Work out the finished part from the listing and answer in its coordinate system (mm). Coordinates: 2 decimals unless noted, no trailing zeros. Write each loop counter-clockwise with the first axis right and the second up, starting at its lowest first coordinate (ties: lowest second). Pieces come first, ordered by that corner, then holes. Notation, with made-up numbers: M 67.5,-26.75 L 97.5,-26.75 A33 cw 97.5,11.25 Z; hole C 39.5,-1.75 d5. An arc over 180 degrees is marked long. Use CSV: the item, a comma, the result in double quotes.
from build123d import *

# Parameters (mm, degrees)
BOSS_EXTRUDE1_DEPTH        = 1.6
F_3_2_3_2_DIAMETER_HOLE3_D = 3.2
FILLET1_R                  = 2


with BuildPart() as part:
    # Sketch1 → Boss-Extrude1 (new body)
    with BuildSketch(Plane.XY):
        with BuildLine():
            Line((-84.56534388, -2.04814307), (-16.56534388, -2.04814307))
            Line((-16.56534388, -2.04814307), (-16.56534388, 7.95185693))
            Line((-16.56534388, 7.95185693), (-6.56534388, 7.95185693))
            Line((-6.56534388, 7.95185693), (-6.56534388, 3.95185693))
            Line((-6.56534388, 3.95185693), (3.425708931, 3.95185693))
            Line((3.425708931, 3.95185693), (3.43465612, 3.95185693))
            ThreePointArc((3.43465612, 3.95185693), (5.555976464, 4.830536587), (6.43465612, 6.95185693))
            Line((6.43465612, 6.95185693), (6.43465612, 88.95185693))
            ThreePointArc((6.43465612, 88.95185693), (5.555976464, 91.073177274), (3.43465612, 91.95185693))
            Line((3.43465612, 91.95185693), (-64.56534388, 91.95185693))
            Line((-64.56534388, 91.95185693), (-64.56534388, 81.95185693))
            Line((-64.56534388, 81.95185693), (-74.56534388, 81.95185693))
            Line((-74.56534388, 81.95185693), (-74.56534388, 85.95185693))
            Line((-74.56534388, 85.95185693), (-84.56534388, 85.95185693))
            ThreePointArc((-84.56534388, 85.95185693), (-86.686664224, 85.073177274), (-87.56534388, 82.95185693))
            Line((-87.56534388, 82.95185693), (-87.56534388, 0.95185693))
            ThreePointArc((-87.56534388, 0.95185693), (-86.686664224, -1.169463413), (-84.56534388, -2.04814307))
        make_face()
    extrude(amount=BOSS_EXTRUDE1_DEPTH)

    # Ø3.2 (3.2) Diameter Hole3 (through all)
    with Locations(Plane(origin=(0, 0, 0), x_dir=(-1, 0, 0), z_dir=(0, 0, -1))):
        with Locations((78.56534388, 6.95185693), (78.56534388, 82.95185693), (2.56534388, 82.95185693), (2.56534388, 6.95185693)):
            Hole(F_3_2_3_2_DIAMETER_HOLE3_D / 2)

    # Fillet1
    fillet1_edges = [part.edges().sort_by_distance(p)[0] for p in [
        (-16.56534388, 7.95185693, 0.8),
        (-74.56534388, 81.95185693, 0.8),
        (-64.56534388, 81.95185693, 0.8),
        (-6.56534388, 7.95185693, 0.8),
    ]]
    fillet(fillet1_edges, radius=FILLET1_R)


solid = part.part
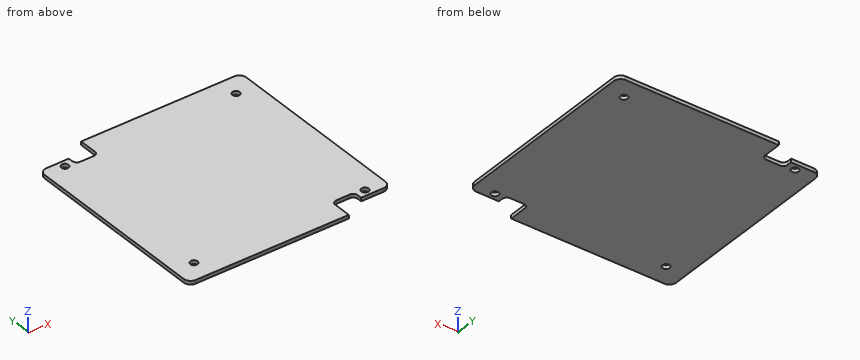
Item 1: The part is cut by section A-A (z = 0.7). Write down the section's boundary in (x, y).
Answer:
outline,"M -87.57,0.95 A3 ccw -84.57,-2.05 L -16.57,-2.05 L -16.57,5.95 A2 cw -14.57,7.95 L -8.57,7.95 A2 cw -6.57,5.95 L -6.57,3.95 L 3.43,3.95 A3 ccw 6.43,6.95 L 6.43,88.95 A3 ccw 3.43,91.95 L -64.57,91.95 L -64.57,83.95 A2 cw -66.57,81.95 L -72.57,81.95 A2 cw -74.57,83.95 L -74.57,85.95 L -84.57,85.95 A3 ccw -87.57,82.95 Z; hole C -78.57,6.95 d3.2; hole C -78.57,82.95 d3.2; hole C -2.57,6.95 d3.2; hole C -2.57,82.95 d3.2"
Item 2: Consider probe 1 along X at (y, z) = (3.5, 1.5); probe 2 along X at (y, z) = (7.5, 1.1); probe 3 along Y at (x, z) = (-3, 1.3). Determine where each line is inside the solid, lowest interval first.
Answer:
probe 1,"x = -87.57 to -16.57"
probe 2,"x = -87.57 to -80.07, -77.06 to -15.83, -7.3 to -4.07, -1.06 to 6.43"
probe 3,"y = 3.95 to 5.41, 8.49 to 81.41, 84.49 to 91.95"
Item 3: Given pin 1 (0.8 mm diameter, centred on x = 1, z = 1, fed in from -Y), flat-ended and moving along its own axis, determine where the tip first touches the part or whether it passes through.
Answer:
pin 1,"stops at y = 3.95"
